The model under review builds one solid part; all positions refer to its coordinate system, in mm. Round coordinates to 2 decimals unless told otherwise and drop trailing zeros. Loops run counter-clockwise (first coordinate to the right, second up) from the corner with the lowest first, then second, coordinate; pieces in that order, holes last. Notation, with made-up numbers: M 66,-23 L 108,-23 A7 cw 108,-15 Z; hole C 27.5,20.25 d8. An arc over 180 degrees is marked long. Return JSON: item names as keys, results as strings. Group by question number.
Q1. Consider section A-A (x = -35). State the section outline as (y, z) points, and give its area (3 significant figures).
Q2. Clearance check with a flat-ended pin moving along its axis: pin 1 Ø5 at (x, y) = (23, 2) entering from -Z. State where the tip first meets the part, or that it passes through.
Q3. To check wall thickness, follow line 1 along Y through (x, z) = (-47.5, 9); line 2 along X through (y, z) = (-0.25, 0.5); line 3 along X through (y, z) = (-1.5, 8.25). State the ranges of each line that lie inside material, in increasing order.
Q4. Consider section C-C (y = -0.25). State the section outline as (x, z) points, and give its area (3 significant figures).
Q5. Consider section B-B (z = 8). State the section outline as (x, y) points, and give its area (3 significant figures).
from build123d import *

# Parameters (mm, degrees)
F1_DEPTH = 15


with BuildPart() as f1:
    # F0 (on Top) → F1 (new body)
    with BuildSketch(Plane.XY):
        Polygon((-55, -2.3), (-55, -5), (55, -5), (55, 5), (-55, 5), (-55, 2.3), (52.3, 2.3), (52.3, -2.3), align=None)
        with BuildLine():
            ThreePointArc((-55, 5), (-60, 0), (-55, -5))
            Line((-55, -5), (-55, -2.3))
            ThreePointArc((-55, -2.3), (-57.3, 0), (-55, 2.3))
            Line((-55, 2.3), (-55, 5))
        make_face()
        with BuildLine():
            ThreePointArc((-55, 2.3), (-57.3, 0), (-55, -2.3))
            Line((-55, -2.3), (-55, 2.3))
        make_face()
    extrude(amount=F1_DEPTH)


solid = f1.part
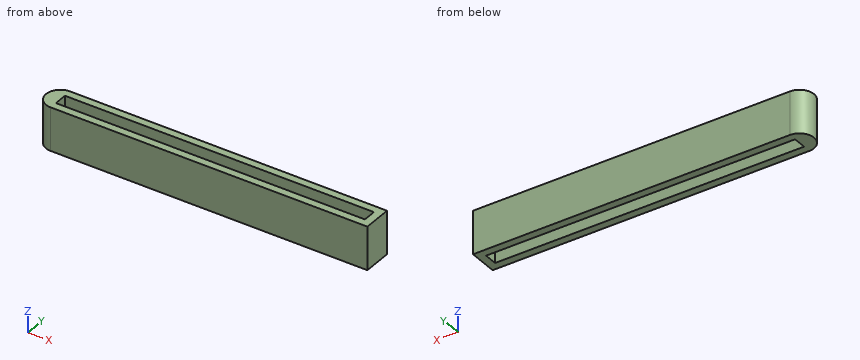
Values:
{
 "1": {"outline": "M -5,0 L -2.3,0 L -2.3,15 L -5,15 Z; M 2.3,0 L 5,0 L 5,15 L 2.3,15 Z", "area": "81.0 mm2"},
 "2": {"pin 1": "stops at z = 0"},
 "3": {"line 1": "y = -5 to -2.3, 2.3 to 5", "line 2": "x = -59.99 to -55, 52.3 to 55", "line 3": "x = -59.77 to -55, 52.3 to 55"},
 "4": {"outline": "M -59.99,0 L -55,0 L -55,15 L -59.99,15 Z; M 52.3,0 L 55,0 L 55,15 L 52.3,15 Z", "area": "115 mm2"},
 "5": {"outline": "M -55,-5 L 55,-5 L 55,5 L -55,5 A5 ccw Z; hole M -55,-2.3 L 52.3,-2.3 L 52.3,2.3 L -55,2.3 Z", "area": "646 mm2"}
}
